```python
from build123d import *

# Parameters (mm, degrees)
SKETCH1_R           = 10
BOSS_EXTRUDE1_DEPTH = 5
FILLET1_R           = 10


with BuildPart() as part:
    # Sketch1 → Boss-Extrude1 (new body)
    with BuildSketch(Plane.XY):
        Polygon((0, -20), (-30, -20), (-30, 40), (-17, 40), (26, 0), (26, -20), align=None)
        Circle(SKETCH1_R, mode=Mode.SUBTRACT)
    extrude(amount=BOSS_EXTRUDE1_DEPTH)

    # Fillet1
    fillet1_edges = [part.edges().sort_by_distance(p)[0] for p in [
        (-17, 40, 2.5),
        (26, 0, 2.5),
        (26, -20, 2.5),
    ]]
    fillet(fillet1_edges, radius=FILLET1_R)


solid = part.part
```
Geometry check sheet. Reference: the model listing, model coordinates, mm. Round coordinates to 2 decimals unless told otherwise and drop trailing zeros. Order: outer loops, then holes, each group sorted by start corner. A loop starts at its lowest first (then second) coordinate and runs counter-clockwise, first axis right, second up. Notation, with made-up numbers: (75, -1) - (83, -1) arc R25 ccw to (83, 24) - close; hole circle Ø1 at (1.25, -0.5). An arc over 180 degrees is marked (long way). Use a Markdown table: item, result. Add a question column.
(1) Sectioned sample at A-A, the plane y = -2. Enter the section's corners in (x, z).
(2) Sectioned sample at C-C, the plane x = 5. Enter the section's corners in (y, z), and give its area (3 significant figures).
(3) Sectioned sample at B-B, the plane z = 0.85. Enter the section's corners in (x, y), and give its area (3 significant figures).
(4) Sectioned sample at D-D, the plane y = 31.5. Enter the section's corners in (x, z), and give its area (3 significant figures).
(5) Material ranges on line 1 along Y through (x, z) = (-7, 0.75); line 2 along X through (y, z) = (5, 3.5) (3 decimals); line 3 along Y through (x, z) = (0, 1.3), recorded low to high. Write a range as [from, to].
(6) Depth check by flat-ended pin: pin 1 (16 mm diameter, centred on x = 0, y = 0, fed in from +Z). Enter the tip coordinate at first touch or a pass-through.
(7) Release check for a two-part mould opening along Y. For faces 1 (the cylindrical face through (25, 0, 3)), 2 (the flat face through (-30, 10, 2)), 3 (the cylindrical face through (22.99, -17.15, 2.54)), 4 (the cylindrical face through (-2.17, -9.76, 2.46)) record: pulls with the +Y half, pulls with the -Y half, needs draft (parallel to the pull), parting line crosses it, or undercut.
Answers below:
| question | item | result |
|---|---|---|
| 1 | outline | (-30, 0) - (-9.8, 0) - (-9.8, 5) - (-30, 5) - close; (9.8, 0) - (25.72, 0) - (25.72, 5) - (9.8, 5) - close |
| 2 | outline | (-20, 0) - (-8.66, 0) - (-8.66, 5) - (-20, 5) - close; (8.66, 0) - (19.53, 0) - (19.53, 5) - (8.66, 5) - close |
| 2 | area | 111 mm² |
| 3 | outline | (-30, -20) - (16, -20) arc R10 ccw to (26, -10) - (26, -4.36) arc R10 ccw to (22.81, 2.97) - (-14.12, 37.32) arc R10 ccw to (-20.93, 40) - (-30, 40) - close; hole circle Ø20 at (0, 0) |
| 3 | area | 2,160 mm² |
| 4 | outline | (-30, 0) - (-7.86, 0) - (-7.86, 5) - (-30, 5) - close |
| 4 | area | 111 mm² |
| 5 | line 1 | [-20, -7.14], [7.14, 30.7] |
| 5 | line 2 | [-30, -8.66], [8.66, 20.625] |
| 5 | line 3 | [-20, -10], [10, 24.19] |
| 6 | pin 1 | through |
| 7 | face 1 | pulls with the +Y half |
| 7 | face 2 | needs draft |
| 7 | face 3 | pulls with the -Y half |
| 7 | face 4 | undercut |
